Autodesk Inventor part; units mm, degrees
ref_plane "Plano de trabajo1" through (2.8, 0, 0) normal (1, 0, 0) x (0, 1, 0)
ref_plane "XZ Plane" through (0, 0, 0) normal (0, 1, 0) x (-1, 0, 0)
ref_plane "XY Plane" through (0, 0, 0) normal (0, 0, 1) x (1, 0, 0)
sketch "Boceto1" plane through (0, 0, 0) normal (1, 0, 0) x (0, 1, 0)
  arc A0 (-2.79, 0) -> (2.79, 0) centre (0, 0) ccw
  line L0 (-2.79, 0) -> (2.79, 0)
  dimension "d0" = 5.58
revolve "Revolución1" add sketch "Boceto1" angle 360 about axis through (0, -2.79, 0) along (0, 1, 0)
ref_plane "Plano de trabajo1" through (2.8, 0, 0) normal (1, 0, 0) x (0, 1, 0)
sketch "Boceto2" plane through (2.8, 0, 0) normal (1, 0, 0) x (0, 1, 0)
  circle A0 centre (0, 0) radius 1.65
  dimension "d3" = 3.3
extrude "Extrusión1" add sketch "Boceto2" along normal blind 1.2 and the other way blind 6.8
sketch "Boceto3" plane through (4, 0, 0) normal (1, 0, 0) x (0, 0, -1)
  circle A0 centre (0, 0) radius 1.65
  circle A1 centre (0, 0) radius 1.25
  dimension "d8" = 2.5
extrude "Extrusión2" cut sketch "Boceto3" against normal blind 13.6 contours A1
fillet "Empalme1" radius 0.08 2 edges at (4, 0, 1.25) (-4, 0, 1.25)
properties part number "Bola_de_libertad_menor" material "Aluminio 6061"
Can you work these out from the model? Positions are in its coordinate system, mm. Give positions to 0.01 mm unless a question says otherwise; leave off trailing zeros. Order: outer loops, then holes, each group sorted by start corner. A loop starts at its lowest first (then second) coordinate and runs counter-clockwise, first axis right, second up. Notation, with made-up numbers: M -14.75,65.25 L 2.25,65.25 A17 ccw 2.25,69.25 Z; hole C 11.5,52.5 d7. An arc over 180 degrees is marked long. Use one line per item in the form item = value. Start each with the question number.
Item 1: If I drill on line 1 along Y through (x, z) = (-1.25, -0.7); line 2 along Y through (x, z) = (1.5, 0); line 3 along Z through (x, y) = (2.75, 0.25), over which ranges is the centre line in solid material (lowest first)?
Item 2: If we section it at C-C (x = 3.25): Write out the boundary of the cut face in (y, z), then the cut area to 3 significant figures.
Item 3: If we section it at D-D (z = -1.5): Write out the boundary of the cut face in (x, y), then the cut area to 3 significant figures.
Item 4: We'd pull the mould along Y, two halves only. Please class faces 1 (the cylindrical face through (3.137, -1.216, 1.115)), 2 (the cylindrical face through (0.05, -1.22, 0.27)): +Y half, -Y half, draft (parallel to the pull), parting line (faces both ways), or undercut.
Item 5: If we section it at A-A (y = 0): Write out the boundary of the cut face in (x, z).
Item 6: Will these pins go through, and if not, where does the flat tip stop? pin 1 Ø2 at (y, z) = (0, 0) entering from +X; pin 2 Ø2 at (x, y) = (0, 2) entering from -Z.
Outcome:
q1.line_1 = -2.39 to -1.04, 1.04 to 2.39
q1.line_2 = -2.35 to -1.25, 1.25 to 2.35
q1.line_3 = -1.63 to -1.22, 1.22 to 1.63
q2.outline = C 0,0 d3.3; hole C 0,0 d2.5
q2.area = 3.64 mm2
q3.outline = M -4,-0.69 L -2.25,-0.69 A2.35 ccw 2.25,-0.69 L 4,-0.69 L 4,0.69 L 2.25,0.69 A2.35 ccw -2.25,0.69 L -4,0.69 Z
q3.area = 22.0 mm2
q4.face_1 = parting line
q4.face_2 = undercut
q5.outline = M -4,-1.65 L -2.25,-1.65 A2.79 ccw 2.25,-1.65 L 4,-1.65 L 4,-1.33 A0.08 ccw 3.92,-1.25 L -3.92,-1.25 A0.08 ccw -4,-1.33 Z; M -4,1.33 A0.08 ccw -3.92,1.25 L 3.92,1.25 A0.08 ccw 4,1.33 L 4,1.65 L 2.25,1.65 A2.79 ccw -2.25,1.65 L -4,1.65 Z
q6.pin_1 = through
q6.pin_2 = -2.6
